Input: part model. Units: mm. Frame: model coordinates. Face numbers are marked on the shaded views. A direction names the side the tool comes from. Give positions to 0.01 mm unless a question says otherwise; leave off trailing zeros. Order: outer loops, then holes, each group sorted by start corner. A loop starts at its lowest first (then second) coordinate and runs counter-clockwise, first axis right, second up.
```python
from build123d import *

# Parameters (mm, degrees)
F1_DEPTH  = 3.175
F4_DEPTH  = 3.175
F6_DEPTH  = 6.35
F7_DEPTH  = 3.175
F9_DEPTH  = 25.4
F11_DEPTH = 3.175
F13_DEPTH = 3.175
F14_DEPTH = 3.175
F15_DEPTH = 6.351


with BuildPart() as f1:
    # F0 (on Top) → F1 (new body)
    with BuildSketch(Plane.XY):
        with BuildLine():
            Line((0, -51.2956328023), (0, -102.09075941))
            ThreePointArc((0, -102.09075941), (72.1890682753, -72.1890682753), (102.09075941, 0))
            Line((102.09075941, 0), (51.2956328023, 0))
            ThreePointArc((51.2956328023, 0), (36.2714897998, -36.2714897998), (0, -51.2956328023))
        make_face()
    extrude(amount=F1_DEPTH)

    # F3 (on face) → F4 (join)
    with BuildSketch(Plane.XY.offset(3.175)):
        with BuildLine():
            ThreePointArc((0, -56.3756328023), (39.8635922482, -39.8635922482), (56.3756328023, 0))
            Line((56.3756328023, 0), (51.3330261441, 0))
            ThreePointArc((51.3330261441, 0), (36.2979308853, -36.2979308853), (0, -51.3330261441))
            Line((0, -51.3330261441), (0, -56.3756328023))
        make_face()
        with BuildLine():
            Line((102.09075941, 0), (97.01075941, 0))
            ThreePointArc((97.01075941, 0), (68.5969658269, -68.5969658269), (0, -97.01075941))
            Line((0, -97.01075941), (0, -102.09075941))
            ThreePointArc((0, -102.09075941), (72.1890682753, -72.1890682753), (102.09075941, 0))
        make_face()
    extrude(amount=F4_DEPTH)

    # F5 (on Top) → F6 (join)
    with BuildSketch(Plane.XY):
        with BuildLine():
            ThreePointArc((54.7619331998, -13.660392724), (56.0189261095, -6.8815386855), (56.4400182242, 0))
            Line((56.4400182242, 0), (51.3051767249, 0))
            ThreePointArc((51.3051767249, 0), (50.8400637591, -6.8926827684), (49.4531579316, -13.660392724))
            Line((49.4531579316, -13.660392724), (54.7619331998, -13.660392724))
        make_face()
        with BuildLine():
            Line((102.1051767249, 0), (97.1390098326, 0))
            ThreePointArc((97.1390098326, 0), (96.8973822865, -6.8472284381), (96.1737017167, -13.660392724))
            Line((96.1737017167, -13.660392724), (101.1872560388, -13.660392724))
            ThreePointArc((101.1872560388, -13.660392724), (101.8754380952, -6.8455990928), (102.1051767249, 0))
        make_face()
    extrude(amount=F6_DEPTH)

    # F2 (on Top) → F7 (join)
    with BuildSketch(Plane.XY):
        Polygon((65.3862244444, -13.4132344524), (65.3862244444, 0.2373858813), (51.3049019501, 0.2373858813), (51.3049019501, -13.4632168472), align=None)
        Polygon((100.5855267867, 0.2373858813), (85.8938746733, 0.2373858813), (85.9641355587, -13.4132344524), (100.5855267867, -13.4132344524), align=None)
    extrude(amount=F7_DEPTH)

    # F8 (on face) → F9 (cut)
    with BuildSketch(Plane.XY.offset(3.175)):
        Polygon((0, -85.8303158734), (13.2304336887, -85.8303158734), (13.2304336887, -79.5142199461), (6.7552071823, -79.5142199461), (3.0578118576, -79.5142199461), (3.0578118576, -71.7228521654), (6.7552071823, -71.7228521654), (13.2304336887, -71.7228521654), (13.2304336887, -65.2524047592), (0, -65.2524047592), align=None)
    extrude(amount=-F9_DEPTH, mode=Mode.SUBTRACT)

    # F10 (on face) → F11 (join)
    with BuildSketch(Plane(origin=(0, 0, 0), x_dir=(1, 0, 0), z_dir=(0, 0, -1))):
        with BuildLine():
            ThreePointArc((39.6434592285, 32.5520826521), (37.980845771, 34.4774897449), (36.2248193412, 36.3181002847))
            Line((36.2248193412, 36.3181002847), (29.0498583475, 29.1246633635))
            Line((29.0498583475, 29.1246633635), (32.646576808, 25.5371828667))
            Line((32.646576808, 25.5371828667), (39.6434592285, 32.5520826521))
        make_face()
        with BuildLine():
            Line((29.0498583475, 29.1246633635), (36.2248193412, 36.3181002847))
            ThreePointArc((36.2248193412, 36.3181002847), (34.3796988436, 38.0693873344), (32.4500223073, 39.7270436459))
            Line((32.4500223073, 39.7270436459), (25.4531398869, 32.7121438604))
            Line((25.4531398869, 32.7121438604), (29.0498583475, 29.1246633635))
        make_face()
        with BuildLine():
            Line((36.2248193412, 36.3181002847), (72.0961827352, 72.2818344532))
            ThreePointArc((72.0961827352, 72.2818344532), (70.2749350461, 74.0537417095), (68.4101530773, 75.7797737714))
            Line((68.4101530773, 75.7797737714), (32.4500223073, 39.7270436459))
            ThreePointArc((32.4500223073, 39.7270436459), (34.3796988436, 38.0693873344), (36.2248193412, 36.3181002847))
        make_face()
        with BuildLine():
            ThreePointArc((75.6035899985, 68.6048127777), (73.8727679087, 70.4651496728), (72.0961827352, 72.2818344532))
            Line((72.0961827352, 72.2818344532), (36.2248193412, 36.3181002847))
            ThreePointArc((36.2248193412, 36.3181002847), (37.980845771, 34.4774897449), (39.6434592285, 32.5520826521))
            Line((39.6434592285, 32.5520826521), (75.6035899985, 68.6048127777))
        make_face()
        with BuildLine():
            Line((79.271143729, 79.4752713743), (72.0961827352, 72.2818344532))
            ThreePointArc((72.0961827352, 72.2818344532), (73.8727679087, 70.4651496728), (75.6035899985, 68.6048127777))
            Line((75.6035899985, 68.6048127777), (82.8785053866, 75.8984614814))
            Line((82.8785053866, 75.8984614814), (79.271143729, 79.4752713743))
        make_face()
        with BuildLine():
            ThreePointArc((68.4101530773, 75.7797737714), (70.2749350461, 74.0537417095), (72.0961827352, 72.2818344532))
            Line((72.0961827352, 72.2818344532), (79.271143729, 79.4752713743))
            Line((79.271143729, 79.4752713743), (75.7328631666, 83.1213402502))
            Line((75.7328631666, 83.1213402502), (68.4101530773, 75.7797737714))
        make_face()
        with BuildLine():
            Line((20.0341812257, 47.2215366883), (40.6881574418, 93.6322433828))
            ThreePointArc((40.6881574418, 93.6322433828), (35.9596571955, 95.5480309127), (31.1413521737, 97.2251991086))
            Line((31.1413521737, 97.2251991086), (10.2418471319, 50.2627746142))
            ThreePointArc((10.2418471319, 50.2627746142), (15.2141958482, 48.9874493037), (20.0341812257, 47.2215366883))
        make_face()
        with BuildLine():
            ThreePointArc((31.1413521737, 97.2251991086), (35.9596571955, 95.5480309127), (40.6881574418, 93.6322433828))
            Line((40.6881574418, 93.6322433828), (44.0618023276, 101.2130230665))
            Line((44.0618023276, 101.2130230665), (34.7585338749, 105.353220427))
            Line((34.7585338749, 105.353220427), (31.1413521737, 97.2251991086))
        make_face()
        with BuildLine():
            Line((16.5176168084, 39.3196083605), (20.0341812257, 47.2215366883))
            ThreePointArc((20.0341812257, 47.2215366883), (15.2141958482, 48.9874493037), (10.2418471319, 50.2627746142))
            Line((10.2418471319, 50.2627746142), (7.7137911807, 44.5820833017))
            Line((7.7137911807, 44.5820833017), (16.5176168084, 39.3196083605))
        make_face()
        with BuildLine():
            ThreePointArc((50.2968928634, 10.0729594896), (49.0339423103, 15.0636796999), (47.2771132537, 19.902675875))
            Line((47.2771132537, 19.902675875), (38.7149937451, 16.3121093065))
            Line((38.7149937451, 16.3121093065), (43.1567628434, 7.0787111473))
            Line((43.1567628434, 7.0787111473), (50.2968928634, 10.0729594896))
        make_face()
        with BuildLine():
            ThreePointArc((97.6098508897, 29.9138791566), (95.9858944102, 34.7740022313), (94.1201154327, 39.5465172658))
            Line((94.1201154327, 39.5465172658), (47.2771132537, 19.902675875))
            ThreePointArc((47.2771132537, 19.902675875), (49.0339423103, 15.0636796999), (50.2968928634, 10.0729594896))
            Line((50.2968928634, 10.0729594896), (97.6098508897, 29.9138791566))
        make_face()
        with BuildLine():
            Line((104.0109246969, 43.6942763627), (94.1201154327, 39.5465172658))
            ThreePointArc((94.1201154327, 39.5465172658), (95.9858944102, 34.7740022313), (97.6098508897, 29.9138791566))
            Line((97.6098508897, 29.9138791566), (107.9681979582, 34.2577025116))
            Line((107.9681979582, 34.2577025116), (104.0109246969, 43.6942763627))
        make_face()
    extrude(amount=F11_DEPTH)

    # F12 (on face) → F13 (join)
    with BuildSketch(Plane(origin=(0, 0, 0), x_dir=(1, 0, 0), z_dir=(0, 0, -1))):
        Polygon((65.3862244444, 0), (65.3862244444, -0.2373858813), (85.8938746733, -0.2373858813), (85.8950965183, 0), align=None)
    extrude(amount=-F13_DEPTH)

    # F14 (add): faces of the model
    f14_faces = [f1.faces().sort_by_distance(p)[0] for p in [
        (67.5252079874, -42.3895565008, 0),
        (42.5870000815, -67.3227346229, 0),
    ]]
    extrude(f14_faces, amount=F14_DEPTH)

    # F2 (on Top) → F15 (cut, through all)
    with BuildSketch(Plane.XY):
        Polygon((79.5788919434, -9.9109848417), (79.5788919434, -6.2948371671), (79.5788919434, 0.2373858813), (71.7875241627, 0.2373858813), (71.7875241627, -6.2948371671), (71.7875241627, -9.9109848417), align=None)
    extrude(amount=F15_DEPTH, mode=Mode.SUBTRACT)


solid = f1.part
```
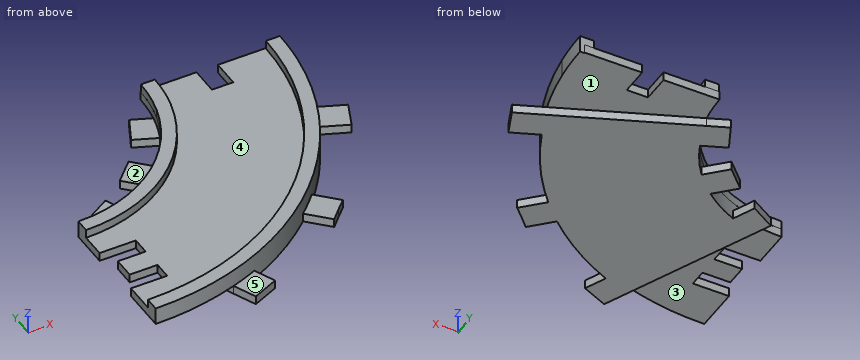
1) First-contact query: P1, Ø1.5, axis at x = 71.5, z = 0, coming from the -Y side; P2, Ø1.5, axis at y = -44.5, z = 3, coming from the -X side; P3, Ø3.5, axis at x = 44, y = -10.5, coming from the +Z side. Flat tips, straight axial feed; report the tip coordinate or a pass-through.
2) Line query: probe 1 along Y at (x, z) = (43, -2.5); probe 2 along Z at (x, y) = (7, -64) (3 decimals); probe 3 along Z at (x, y) = (66.5, -22) (3 decimals). Output: solid intervals per line, ascending.
3) Cut plane D-D (x = 60). Return the cut outline in (y, z) (3 decimals).
4) Cut plane B-B (y = -27.5). Return the cut outline in (x, z) (3 decimals).
5) Pull-direction query (Y, two-part tool) for the marked faces 4 and 5; classes: pulls with the +Y half, pulls with the -Y half, needs draft (parallel to the pull), parting line crosses it, or undercut.
6) Cut plane C-C (z = -1.75). Return the cut outline in (x, y) (1 decimal).
7) Reachability of the marked faces 1, 2 and 3 from +Z, -Z, +X, -X, +Y, -Y: full face, straight path, thin tool, end or side. Return the list, or none.
Geometry says:
1. P1: stops at y = -79.63
1. P2: stops at x = 24.16
1. P3: stops at z = 0
2. probe 1: y = -101.69 to -98.83, -92.59 to -27.97, -18.11 to -7.4
2. probe 2: z = 0 to 3.175
2. probe 3: z = -3.175 to 3.175
3. outline: (-82.599, -3.175) - (-14.142, -3.175) - (-14.142, 0) - (0.237, 0) - (0.237, 3.175) - (-76.23, 3.175) - (-76.23, 6.35) - (-82.599, 6.35) - close
4. outline: (30.679, -3.175) - (34.604, -3.175) - (34.604, 0) - (30.679, 0) - close; (43.301, -3.175) - (91.854, -3.175) - (91.854, 0) - (98.317, 0) - (98.317, 6.35) - (93.031, 6.35) - (93.031, 3.175) - (49.213, 3.175) - (49.213, 6.35) - (43.345, 6.35) - (43.345, 3.175) - (43.301, 3.175) - close
5. face 4: undercut
5. face 5: needs draft
6. outline: (7.7, -44.6) - (34.8, -105.4) - (44.1, -101.2) - (40.7, -93.6) arc R102.1 ccw to (68.4, -75.8) - (75.7, -83.1) - (79.3, -79.5) - (82.9, -75.9) - (75.6, -68.6) arc R102.1 ccw to (94.1, -39.5) - (104, -43.7) - (108, -34.3) - (43.2, -7.1) - (38.7, -16.3) - (47.3, -19.9) arc R51.3 cw to (39.6, -32.6) - (32.6, -25.5) - (25.5, -32.7) - (32.5, -39.7) arc R51.3 cw to (20, -47.2) - (16.5, -39.3) - close
7. face 1: -Z, +X, +Y
7. face 2: +Z, -X, +Y
7. face 3: -Z, -X, -Y
